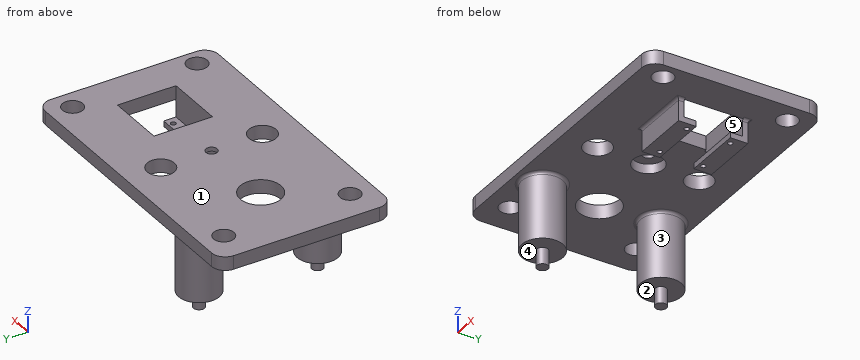
```python
from build123d import *

# Parameters (mm, degrees)
SKETCH1_W            = 216
SKETCH1_H            = 127
BOSS_EXTRUDE1_DEPTH  = 10
FILLET1_R            = 10
FILLET2_R            = 10
SKETCH9_R            = 11.15
CUT_EXTRUDE4_DEPTH   = 7
SKETCH12_R           = 4.15
CUT_EXTRUDE5_DEPTH   = 7
SKETCH9_4_W          = 43
SKETCH9_4_H          = 43
CUT_EXTRUDE6_DEPTH   = 126.683133315
SKETCH13_W           = 43
SKETCH13_H           = 4
BOSS_EXTRUDE2_DEPTH  = 17
FILLET4_R            = 2
SKETCH17_W           = 43
SKETCH17_H           = 4
BOSS_EXTRUDE5_DEPTH  = 9
SKETCH18_W           = 43
SKETCH18_H           = 4
BOSS_EXTRUDE6_DEPTH  = 17
SKETCH19_W           = 43
SKETCH19_H           = 4
BOSS_EXTRUDE7_DEPTH  = 9
FILLET5_R            = 2
SKETCH20_R           = 1.85
CUT_EXTRUDE7_DEPTH   = 9
SKETCH23_R           = 1.85
CUT_EXTRUDE8_DEPTH   = 9
SKETCH25_R           = 15
BOSS_EXTRUDE9_DEPTH  = 48.84
SKETCH26_R           = 4.15
BOSS_EXTRUDE10_DEPTH = 12
SKETCH27_R           = 4.15
BOSS_EXTRUDE11_DEPTH = 12
FILLET9_R            = 2
FILLET10_R           = 2
SKETCH28_R           = 7.5
CUT_EXTRUDE9_DEPTH   = 144.925521017
SKETCH29_R           = 15
SKETCH29_R_2         = 10
CUT_EXTRUDE10_DEPTH  = 140.275825612


with BuildPart() as part:
    # Sketch1 → Boss-Extrude1 (new body)
    with BuildSketch(Plane.XY):
        Rectangle(SKETCH1_W, SKETCH1_H)
    extrude(amount=BOSS_EXTRUDE1_DEPTH)

    # Fillet1
    fillet1_edges = [part.edges().sort_by_distance(p)[0] for p in [
        (-108, 63.5, 5),
    ]]
    fillet(fillet1_edges, radius=FILLET1_R)

    # Fillet2
    fillet2_edges = [part.edges().sort_by_distance(p)[0] for p in [
        (108, -63.5, 5),
        (-108, -63.5, 5),
        (108, 63.5, 5),
    ]]
    fillet(fillet2_edges, radius=FILLET2_R)

    # Sketch9 → Cut-Extrude4 (cut)
    with BuildSketch(Plane(origin=(0, 0, 0), x_dir=(-1, 0, 0), z_dir=(0, 0, -1))):
        with Locations((-4, 0)):
            Circle(SKETCH9_R)
    extrude(amount=-CUT_EXTRUDE4_DEPTH, mode=Mode.SUBTRACT)

    # Sketch12 → Cut-Extrude5 (cut)
    with BuildSketch(Plane(origin=(0, 0, 7), x_dir=(-1, 0, 0), z_dir=(0, 0, -1))):
        with Locations((-4, 0)):
            Circle(SKETCH12_R)
    extrude(amount=-CUT_EXTRUDE5_DEPTH, mode=Mode.SUBTRACT)

    # Sketch9_4 → Cut-Extrude6 (cut, through all)
    with BuildSketch(Plane(origin=(0, 0, 0), x_dir=(-1, 0, 0), z_dir=(0, 0, -1))):
        with Locations((-59, 0)):
            Rectangle(SKETCH9_4_W, SKETCH9_4_H)
    extrude(amount=-CUT_EXTRUDE6_DEPTH, mode=Mode.SUBTRACT)

    # Sketch13 → Boss-Extrude2 (add)
    with BuildSketch(Plane(origin=(0, 0, 0), x_dir=(-1, 0, 0), z_dir=(0, 0, -1))):
        with Locations((-59, -23.5)):
            Rectangle(SKETCH13_W, SKETCH13_H)
    extrude(amount=BOSS_EXTRUDE2_DEPTH)

    # Fillet4
    fillet4_edges = [part.edges().sort_by_distance(p)[0] for p in [
        (37.5, -23.5, 0),
        (80.5, -23.5, 0),
        (59, -25.5, 0),
    ]]
    fillet(fillet4_edges, radius=FILLET4_R)

    # Sketch17 → Boss-Extrude5 (add)
    with BuildSketch(Plane(origin=(0, -21.5, 0), x_dir=(1, 0, 0), z_dir=(0, 1, 0))):
        with Locations((59, 15)):
            Rectangle(SKETCH17_W, SKETCH17_H)
    extrude(amount=BOSS_EXTRUDE5_DEPTH)

    # Sketch18 → Boss-Extrude6 (add)
    with BuildSketch(Plane(origin=(0, 0, 0), x_dir=(-1, 0, 0), z_dir=(0, 0, -1))):
        with Locations((-59, 23.5)):
            Rectangle(SKETCH18_W, SKETCH18_H)
    extrude(amount=BOSS_EXTRUDE6_DEPTH)

    # Sketch19 → Boss-Extrude7 (add)
    with BuildSketch(Plane(origin=(0, 21.5, 0), x_dir=(-1, 0, 0), z_dir=(0, -1, 0))):
        with Locations((-59, 15)):
            Rectangle(SKETCH19_W, SKETCH19_H)
    extrude(amount=BOSS_EXTRUDE7_DEPTH)

    # Fillet5
    fillet5_edges = [part.edges().sort_by_distance(p)[0] for p in [
        (37.5, 23.5, 0),
        (59, 25.5, 0),
        (80.5, 23.5, 0),
    ]]
    fillet(fillet5_edges, radius=FILLET5_R)

    # Sketch20 → Cut-Extrude7 (cut)
    with BuildSketch(Plane(origin=(0, 0, -17), x_dir=(-1, 0, 0), z_dir=(0, 0, -1))):
        with Locations((-43.15, -16)):
            Circle(SKETCH20_R)
        with Locations((-74.85, -16)):
            Circle(SKETCH20_R)
    extrude(amount=-CUT_EXTRUDE7_DEPTH, mode=Mode.SUBTRACT)

    # Sketch23 → Cut-Extrude8 (cut)
    with BuildSketch(Plane(origin=(0, 0, -17), x_dir=(-1, 0, 0), z_dir=(0, 0, -1))):
        with Locations((-43.15, 15.85)):
            Circle(SKETCH23_R)
        with Locations((-74.85, 16)):
            Circle(SKETCH23_R)
    extrude(amount=-CUT_EXTRUDE8_DEPTH, mode=Mode.SUBTRACT)

    # Sketch25 → Boss-Extrude9 (add)
    with BuildSketch(Plane(origin=(0, 0, 0), x_dir=(-1, 0, 0), z_dir=(0, 0, -1))):
        with Locations(Location((51.068737931, -43.5, 0), (0, 0, 180))):
            Circle(SKETCH25_R)
        with Locations(Location((51.068737931, 43.5, 0), (0, 0, 180))):
            Circle(SKETCH25_R)
    extrude(amount=BOSS_EXTRUDE9_DEPTH)

    # Sketch26 → Boss-Extrude10 (add)
    with BuildSketch(Plane(origin=(0, 0, -48.84), x_dir=(-1, 0, 0), z_dir=(0, 0, -1))):
        with Locations((51.068737931, -43.5)):
            Circle(SKETCH26_R)
    extrude(amount=BOSS_EXTRUDE10_DEPTH)

    # Sketch27 → Boss-Extrude11 (add)
    with BuildSketch(Plane(origin=(0, 0, -48.84), x_dir=(-1, 0, 0), z_dir=(0, 0, -1))):
        with Locations((51.068737931, 43.5)):
            Circle(SKETCH27_R)
    extrude(amount=BOSS_EXTRUDE11_DEPTH)

    # Fillet9
    fillet9_edges = [part.edges().sort_by_distance(p)[0] for p in [
        (-66.068737931, -43.5, 0),
    ]]
    fillet(fillet9_edges, radius=FILLET9_R)

    # Fillet10
    fillet10_edges = [part.edges().sort_by_distance(p)[0] for p in [
        (-66.068737931, 43.5, 0),
    ]]
    fillet(fillet10_edges, radius=FILLET10_R)

    # Sketch28 → Cut-Extrude9 (cut, through all)
    with BuildSketch(Plane.XY.offset(10)):
        with Locations((-84.811667967, 46.37)):
            Circle(SKETCH28_R)
        with Locations((-84.811667967, -46.37)):
            Circle(SKETCH28_R)
        with Locations((95.674047271, -46.369786546)):
            Circle(SKETCH28_R)
        with Locations((93.399057455, 46.37)):
            Circle(SKETCH28_R)
    extrude(amount=-CUT_EXTRUDE9_DEPTH, mode=Mode.SUBTRACT)

    # Sketch29 → Cut-Extrude10 (cut, through all)
    with BuildSketch(Plane(origin=(0, 0, 0), x_dir=(-1, 0, 0), z_dir=(0, 0, -1))):
        with Locations((53.828265838, 0)):
            Circle(SKETCH29_R)
        with Locations((-4, -37.325)):
            Circle(SKETCH29_R_2)
        with Locations((-4, 37.325)):
            Circle(SKETCH29_R_2)
    extrude(amount=-CUT_EXTRUDE10_DEPTH, mode=Mode.SUBTRACT)


solid = part.part
```
Model file for the job. Use its own axes, mm. Face numbers are marked on the shaded views. A direction names the side the tool comes from. Coordinates: 2 decimals unless noted, no trailing zeros. Loops run counter-clockwise (first coordinate to the right, second up) from the corner with the lowest first, then second, coordinate; pieces in that order, holes last. Notation, with made-up numbers: M -15.75,53.5 L -8.75,53.5 A29 ccw -8.75,73.5 Z; hole C 64,38 d7. An arc over 180 degrees is marked long. Use CSV: the item, a comma, the result in double quotes. Start each with the question number.
1. Band-saw the part on A-A, the plane x = 4. List the corners of the cut face in (y, z) (3 decimals), then the cut area to 3 significant figures.
2. Band-saw the part on B-B, the plane z = -8.5. List the corners of the cut face in (x, y), then the cut area to 3 significant figures.
3. Tool access for the marked faces 1 and 2: list every direction of +Z, -Z, +X, -X, +Y, -Y with a clear straight run to the whole face (end or side of a thin tool).
4. Band-saw the part on D-D, the plane x = 64. List the corners of the cut face in (y, z), then the cut area to 3 significant figures.
5. Flat gauge pins, fed straight in: pin 1 (12 mm diameter, centred on y = 50.5, z = -26.5, fed in from -X); pin 2 (6.5 mm diameter, centred on x = 4, y = 0, fed in from -Z); pin 3 (11 mm diameter, centred on x = 5.5, y = -1, fed in from -Z); pin 4 (8 mm diameter, centred on x = 41, z = -17, fed in from +Y). Where does each tip first touch, or does it go through?
6. Two-plate mould, pull along X, no slides. Class the marked faces 3, 4 and 5: pulls with the +X half, pulls with the -X half, needs draft (parallel to the pull), parting line crosses it, or undercut.
7. Band-saw the part on C-C, the plane y = -43.5. List the corners of the cut face in (x, z), then the cut area to 3 significant figures.
8. Probe probe 1 along X at (y, z) = (-12, 0.5); probe 2 along Y at (x, z) = (4, 3) (3 decimals); probe 3 along Y at (x, z) = (-78, 3.5). List the from-to ranges inside material, lowest first. Write a range as [from, to].
Entries:
1,outline,"M -63.5,0 L -47.325,0 L -47.325,10 L -63.5,10 Z; M -27.325,0 L -11.15,0 L -11.15,7 L -4.15,7 L -4.15,10 L -27.325,10 Z; M 4.15,7 L 11.15,7 L 11.15,0 L 27.325,0 L 27.325,10 L 4.15,10 Z; M 47.325,0 L 63.5,0 L 63.5,10 L 47.325,10 Z"
1,area,"689 mm2"
2,outline,"C -51.07,-43.5 d30; C -51.07,43.5 d30; M 37.5,-25.5 L 80.5,-25.5 L 80.5,-21.5 L 37.5,-21.5 Z; M 37.5,21.5 L 80.5,21.5 L 80.5,25.5 L 37.5,25.5 Z"
2,area,"1,760 mm2"
3,face 1,"+Z, +X, -X, +Y, -Y"
3,face 2,"-Z"
4,outline,"M -63.5,0 L -27.5,0 A2 cw -25.5,-2 L -25.5,-17 L -12.5,-17 L -12.5,-13 L -21.5,-13 L -21.5,10 L -63.5,10 Z; M 12.5,-17 L 25.5,-17 L 25.5,-2 A2 cw 27.5,0 L 63.5,0 L 63.5,10 L 21.5,10 L 21.5,-13 L 12.5,-13 Z"
4,area,"1,050 mm2"
5,pin 1,"stops at x = -66.04"
5,pin 2,"passes through"
5,pin 3,"stops at z = 7"
5,pin 4,"stops at y = 25.5"
6,face 3,"parting line crosses it"
6,face 4,"needs draft"
6,face 5,"undercut"
7,outline,"M -108,0 L -91.74,0 L -91.74,10 L -108,10 Z; M -77.88,0 L -68.07,0 A2 cw -66.07,-2 L -66.07,-48.84 L -55.22,-48.84 L -55.22,-60.84 L -46.92,-60.84 L -46.92,-48.84 L -36.07,-48.84 L -36.07,-2 A2 cw -34.07,0 L -3.87,0 L -3.87,10 L -77.88,10 Z; M 11.87,0 L 88.74,0 L 88.74,10 L 11.87,10 Z; M 102.6,0 L 108,0 L 108,10 L 102.6,10 Z"
7,area,"3,290 mm2"
8,probe 1,"x = [-108, -62.83], [-44.83, 37.5], [80.5, 108]"
8,probe 2,"y = [-63.5, -47.325], [-27.325, -11.15], [11.15, 27.325], [47.325, 63.5]"
8,probe 3,"y = [-63.5, -49.51], [-43.23, 43.23], [49.51, 63.5]"
